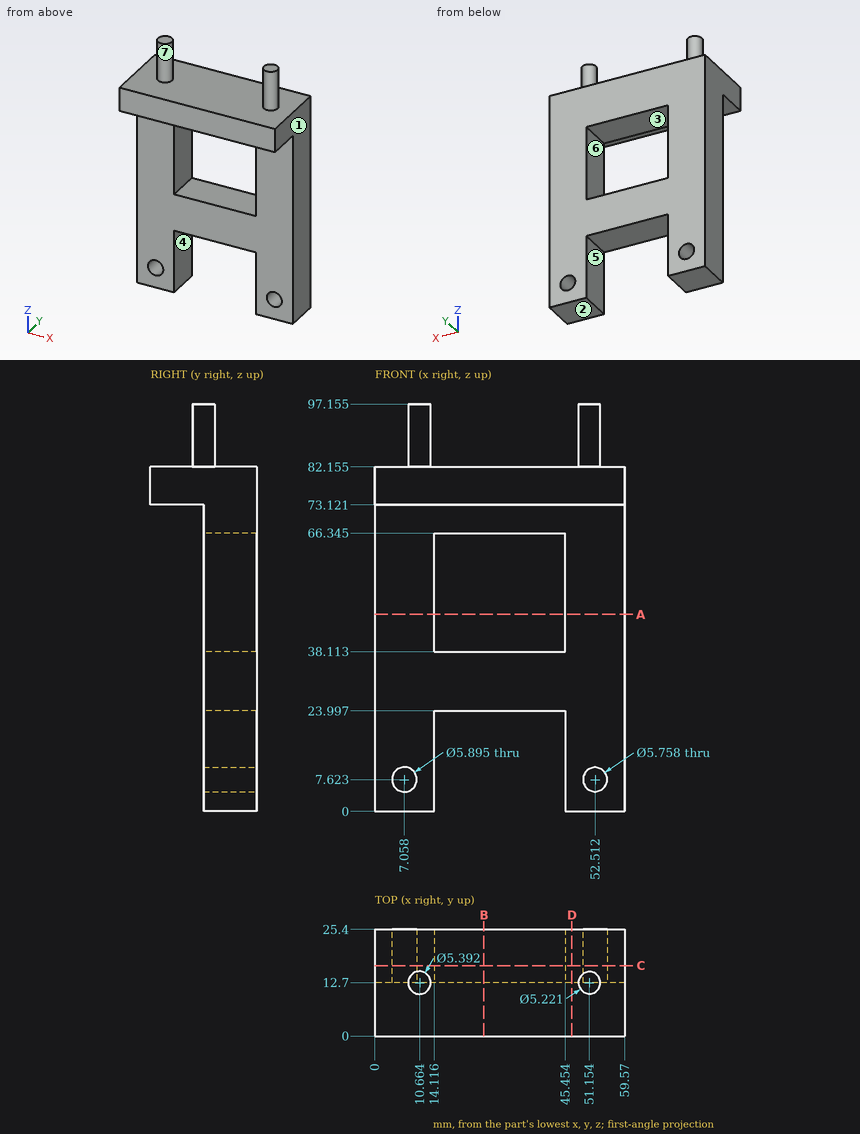
Geometry check sheet. Reference: drawing and pictorial views, mm from the part's lowest x, y, z. A direction names the side the tool comes from. Coordinates: 2 decimals unless noted, no trailing zeros. Order: outer loops, then holes, each group sorted by start corner. A loop starts at its lowest first (then second) coordinate and runs counter-clockwise, first axis right, second up. Notation, with made-up numbers: M -33.75,22 L 6.25,22 A10 ccw 6.25,38 Z; hole C 67.25,-1.75 d11. An arc over 180 degrees is marked long. Write each question's results on one line, items separated by ' | '. Start each with the question number.
1. Cross-section at A-A on z = 47. Record the cut outline in (x, y).
2. Mould release check, pull along X, two halves, no side actions. Record for the marked faces 1, 2, 3 and 4: +X half, -X half, draft (parallel to the pull), parting line (faces both ways), or undercut.
3. Cross-section at D-D on x = 47. Record the cut outline in (y, z) (1 decimal).
4. Go/stop test with flat-tipped pins: P1, Ø6.5, axis at y = 18, z = 15.5, coming from the -X side; P2, Ø4, axis at x = 23.5, y = 18.5, coming from the +Z side (1 decimal); P3, Ø1, axis at x = 37.5, y = 7, coming from the -Z side; P4, Ø6.5, axis at x = 26.5, y = 20, coming from the -Z side. Record where each tip stops, or that it passes through.
5. Material ranges on probe 1 along Z at (x, y) = (22.5, 23) (1 decimal); probe 2 along X at (y, z) = (23.25, 7) (1 decimal); probe 3 along X at (y, z) = (14.5, 50.5), recorded low to high.
6. Access from +Z, -Z, +X, -X, +Y, -Y to the whole of each face (thin tool, end or side, straight path). Record for the marked faces 5, 6 and 7.
7. Cross-section at C-C on y = 16.75. Record the cut outline in (x, z) (1 decimal), and give its area (3 significant figures).
8. Cross-section at B-B on x = 26. Record the cut outline in (y, z) (1 decimal), and give its area (3 significant figures).
Checks:
1) outline: M 0,12.7 L 14.12,12.7 L 14.12,25.4 L 0,25.4 Z; M 45.45,12.7 L 59.57,12.7 L 59.57,25.4 L 45.45,25.4 Z
2) face 1: +X half | face 2: draft | face 3: undercut | face 4: undercut
3) outline: M 0,73.1 L 12.7,73.1 L 12.7,0 L 25.4,0 L 25.4,82.2 L 0,82.2 Z
4) P1: stops at x = 0 | P2: stops at z = 82.2 | P3: stops at z = 73.12 | P4: stops at z = 24
5) probe 1: z = 24 to 38.1, 66.3 to 82.2 | probe 2: x = 0 to 4.2, 9.9 to 14.1, 45.5 to 49.7, 55.3 to 59.6 | probe 3: x = 0 to 14.12, 45.45 to 59.57
6) face 5: -Z, +Y, -Y | face 6: +Y, -Y | face 7: +Z
7) outline: M 0,0 L 14.1,0 L 14.1,24 L 45.5,24 L 45.5,0 L 59.6,0 L 59.6,82.2 L 0,82.2 Z; hole C 7.1,7.6 d5.9; hole M 14.1,38.1 L 45.5,38.1 L 45.5,66.3 L 14.1,66.3 Z; hole C 52.5,7.6 d5.8 | area: 3,200 mm²
8) outline: M 0,73.1 L 12.7,73.1 L 12.7,66.3 L 25.4,66.3 L 25.4,82.2 L 0,82.2 Z; M 12.7,24 L 25.4,24 L 25.4,38.1 L 12.7,38.1 Z | area: 495 mm²
